from build123d import *

# Parameters (mm, degrees)
SKETCH1_W          = 3
SKETCH1_H          = 8
SKETCH1_W_2        = 10
SKETCH1_H_2        = 4
SKETCH2_R          = 2.5
CUT_EXTRUDE1_DEPTH = 36


with BuildPart() as part:
    # Sketch1 → Revolve2 (revolve)
    with BuildSketch(Plane(origin=(0, 0, 0), x_dir=(1, 0, 0), z_dir=(0, 1, 0))):
        Polygon((3.5, 0), (-3.5, 0), (-3.5, -10), (3.5, -10), (3.5, -8), align=None)
        with Locations((5, -4)):
            Rectangle(SKETCH1_W, SKETCH1_H)
        Polygon((24.5, 0), (6.5, 0), (6.5, -8), (6.5, -13), (24.5, -13), (24.5, -10), align=None)
        Polygon((38.5, 0), (24.5, 0), (24.5, -10), (38.5, -10), (38.5, -8), align=None)
        Polygon((51.5, 0), (38.5, 0), (38.5, -8), (51.5, -8), (51.5, -6), align=None)
        Polygon((68.5, 0), (51.5, 0), (51.5, -6), (68.5, -6), (68.5, -4), align=None)
        with Locations((73.5, -2)):
            Rectangle(SKETCH1_W_2, SKETCH1_H_2)
    revolve(axis=Axis((-3.5, 0, 0), (1, 0, 0)))

    # Sketch2 → Cut-Extrude1 (cut)
    with BuildSketch(Plane.ZY.offset(3.5)):
        Circle(SKETCH2_R)
    extrude(amount=-CUT_EXTRUDE1_DEPTH, mode=Mode.SUBTRACT)

    # Sketch3 → Cut-Revolve2 (revolve, cut)
    with BuildSketch(Plane.XY):
        Polygon((32.5, 0), (34.5, 0), (32.5, -2.5), align=None)
    revolve(axis=Axis((34.5, 0, 0), (-1, 0, 0)), mode=Mode.SUBTRACT)


solid = part.part
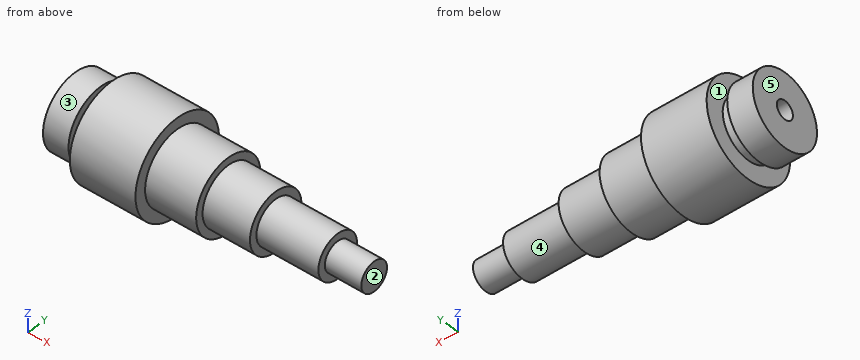
CAD build for the part. Positions are in the model's coordinates, mm. Face numbers are marked on the shaded views. A direction names the side the tool comes from. Give positions to 0.01 mm unless a question says otherwise; leave off trailing zeros. Write each loop counter-clockwise with the first axis right and the second up, starting at its lowest first coordinate (ties: lowest second). Pieces come first, ordered by that corner, then holes. Notation, with made-up numbers: (73, 36.5) -> (131, 36.5) arc R29 cw to (131, 70.5) -> close; hole circle Ø8 at (30.25, 48.5). An arc over 180 degrees is marked (long way). Return JSON: item names as keys, results as strings.
Item 1: Band-saw the part on C-C (x = 35.5). List the corners of the cut face in (y, z), then the cut area to 3 significant figures.
Answer below:
{"outline": "circle Ø20 at (0, 0)", "area": "314 mm2"}
Item 2: Band-saw the part on A-A (x = 8.5). List the corners of the cut face in (y, z).
Answer below:
{"outline": "circle Ø26 at (0, 0); hole circle Ø5 at (0, 0)"}
Item 3: Tool access for the marked faces 4 and 5: list every direction of +Z, -Z, +X, -X, +Y, -Y with a clear straight run to the whole face (end or side of a thin tool).
Answer below:
{"face 4": "+X", "face 5": "+Z, -Z, -X, +Y, -Y"}
Item 4: Drop flat-ended pins along their axis: pin 1 (6 mm diameter, centred on x = 46, z = 0.5, fed in from -Y); pin 2 (4 mm diameter, centred on y = 8.5, z = 0.5, fed in from +X); pin 3 (1 mm diameter, centred on x = 43, z = -6, fed in from +Y). Give the stop position or say it passes through.
Answer below:
{"pin 1": "stops at y = -8", "pin 2": "stops at x = 51.5", "pin 3": "stops at y = 5.81"}
Item 5: Two-plate mould, pull along X, no slides. Class the marked faces 1, 2 and 3: +X half, -X half, draft (parallel to the pull), parting line (faces both ways), or undercut.
Answer below:
{"face 1": "undercut", "face 2": "+X half", "face 3": "draft"}
Item 6: Band-saw the part on B-B (z = -3.25). List the corners of the cut face in (x, y), then the cut area to 3 significant figures.
Answer below:
{"outline": "(-3.5, -9.46) -> (3.5, -9.46) -> (3.5, -7.31) -> (6.5, -7.31) -> (6.5, -12.59) -> (24.5, -12.59) -> (24.5, -9.46) -> (38.5, -9.46) -> (38.5, -7.31) -> (51.5, -7.31) -> (51.5, -5.04) -> (68.5, -5.04) -> (68.5, -2.33) -> (78.5, -2.33) -> (78.5, 2.33) -> (68.5, 2.33) -> (68.5, 5.04) -> (51.5, 5.04) -> (51.5, 7.31) -> (38.5, 7.31) -> (38.5, 9.46) -> (24.5, 9.46) -> (24.5, 12.59) -> (6.5, 12.59) -> (6.5, 7.31) -> (3.5, 7.31) -> (3.5, 9.46) -> (-3.5, 9.46) -> close", "area": "1,300 mm2"}
Item 7: Band-saw the part on D-D (x = 72). List the corners of the cut face in (y, z).
Answer below:
{"outline": "circle Ø8 at (0, 0)"}
Item 8: Drill centre lines: probe 1 along Y at (x, z) = (19.5, 0); probe 2 along X at (y, z) = (7, 1.25). Where is each one in solid material? Low to high.
Answer below:
{"probe 1": "y = -13 to -2.5, 2.5 to 13", "probe 2": "x = -3.5 to 51.5"}
